Read the model definition and answer for the solid it produces. Units are mm, in the model's axes. Face numbers are marked on the shaded views. A direction names the side the tool comes from. Coordinates: 2 decimals unless noted, no trailing zeros. Loops run counter-clockwise (first coordinate to the right, second up) from the corner with the lowest first, then second, coordinate; pieces in that order, holes last.
from build123d import *

# Parameters (mm, degrees)
CUT_EXTRUDE1_REACH = 32.904


with BuildPart() as part:
    # Sketch1 → Revolve1 (revolve)
    with BuildSketch(Plane(origin=(0, 0, 0), x_dir=(0, 0, -1), z_dir=(1, 0, 0)), mode=Mode.PRIVATE) as revolve1_sk:
        with BuildLine():
            Line((-5.08, 20.6375), (5.08, 20.6375))
            Line((5.08, 20.6375), (5.08, 13.716))
            ThreePointArc((5.08, 13.716), (4.064, 12.7), (5.08, 11.684))
            Line((5.08, 11.684), (5.08, 0))
            Line((5.08, 0), (-5.08, 0))
            Line((-5.08, 0), (-5.08, 11.684))
            ThreePointArc((-5.08, 11.684), (-4.064, 12.7), (-5.08, 13.716))
            Line((-5.08, 13.716), (-5.08, 20.6375))
        make_face()
    revolve(revolve1_sk.sketch.rotate(Axis((0, 0, 5.08), (0, 0, -1)), 90), axis=Axis((0, 0, 5.08), (0, 0, -1)))

    # Sketch2 → Cut-Extrude1 (cut, up to next)
    with BuildSketch(Plane.XY.offset(5.08), mode=Mode.PRIVATE) as cut_extrude1_sk1:
        Polygon((-3.666174209, 6.35), (-7.332348419, 0), (-3.666174209, -6.35), (3.666174209, -6.35), (7.332348419, 0), (3.666174209, 6.35), align=None)
    cut_extrude1_tool1 = extrude(cut_extrude1_sk1.sketch, amount=-CUT_EXTRUDE1_REACH, mode=Mode.PRIVATE) & part.part
    add(cut_extrude1_tool1.solids().sort_by_distance((0, 0, 5.08))[0], mode=Mode.SUBTRACT)


solid = part.part
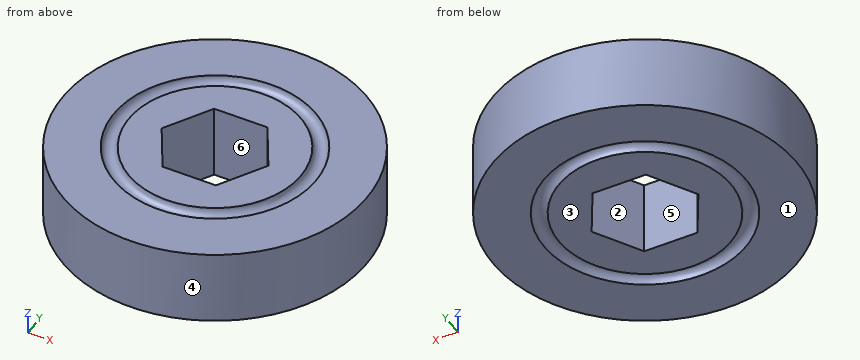
Q1. Straight lines are drawn through the part: probe 1 along Y at (x, z) = (1, -4.25); probe 2 along Y at (x, z) = (8.5, 4.5); probe 3 along Y at (x, z) = (-2, 0.75). For each, find the intervals that lie inside material, in ascending order.
Findings below:
probe 1: y = -20.61 to -13.25, -12.07 to -6.35, 6.35 to 12.07, 13.25 to 20.61
probe 2: y = -18.81 to -10.53, -8.28 to 8.28, 10.53 to 18.81
probe 3: y = -20.54 to -6.35, 6.35 to 20.54
Q2. Which of the six approach directions +Z, -Z, +X, -X, +Y, -Y give full straight-line access (tool end or side, diameter ignored) to the marked faces 1 and 2?
Findings below:
face 1: -Z, +X, -X, +Y, -Y
face 2: +Z, -Z
Q3. A cutting plane is placed at A-A (x = 0). Give the vertices of the cut face in (y, z), then the cut area to 3 significant figures.
Findings below:
outline: (-20.64, -5.08) - (-13.72, -5.08) arc R1.02 cw to (-11.68, -5.08) - (-6.35, -5.08) - (-6.35, 5.08) - (-11.68, 5.08) arc R1.02 cw to (-13.72, 5.08) - (-20.64, 5.08) - close; (6.35, -5.08) - (11.68, -5.08) arc R1.02 cw to (13.72, -5.08) - (20.64, -5.08) - (20.64, 5.08) - (13.72, 5.08) arc R1.02 cw to (11.68, 5.08) - (6.35, 5.08) - close
area: 284 mm2
Q4. Flat-ended cylindrical pins translate along their axes: pin 1 Ø1.5 at (x, z) = (-11, -4) entering from +Y; pin 2 Ø6 at (x, z) = (1.5, -2) entering from +Y; pin 3 Ø1 at (y, z) = (15, 1.5) entering from -X. Find the tip coordinate at first contact, or state that the pin passes through.
Findings below:
pin 1: stops at y = 17.91
pin 2: stops at y = 20.64
pin 3: stops at x = -14.69
Q5. Determine the mould class of the marked faces 3, 4, 5 and 6 for opening direction X: +X half, -X half, draft (parallel to the pull), parting line (faces both ways), or undercut.
Findings below:
face 3: draft
face 4: parting line
face 5: undercut
face 6: undercut
